Autodesk Inventor part; units mm, degrees
ref_plane "YZ Plane" through (0, 0, 0) normal (1, 0, 0) x (0, 1, 0)
ref_plane "XY Plane" through (0, 0, 0) normal (0, 0, 1) x (1, 0, 0)
sketch "Sketch1" plane through (0, 0, 0) normal (0, 0, 1) x (1, 0, 0)
  circle A0 centre (0, 0) radius 2.159
  dimension "d0" = 4.318
extrude "Extrusion1" add sketch "Sketch1" along normal blind 8.128
sketch "Sketch2" plane through (0, 0, 0) normal (0, 0, -1) x (-1, 0, 0)
  circle A0 centre (0, 0) radius 2.159
  circle A1 centre (0, 0) radius 1.4986
  dimension "d3" = 2.9972
extrude "Extrusion2" cut sketch "Sketch2" against normal blind 6.096
sketch "Sketch3" plane through (0, 0, 0) normal (0, 1, 0) x (-1, 0, 0)
  line L0 (-2.159, 8.128) -> (2.159, 8.128)
  line L1 (0, -2.8448) -> (0, 17.0688)
  line L2 (2.159, 8.128) -> (0, 8.128)
  line L3 (0, 8.128) -> (0, 14.478)
  line L4 (2.159, 6.096) -> (-2.159, 6.096)
  line L5 (-2.159, 8.128) -> (2.159, 8.128)
  line L6 (2.159, 6.096) -> (2.159, 8.128)
  line L7 (-1.4986, 0) -> (1.4986, 0)
  line L8 (0, 14.478) -> (1.9685, 14.478)
  line L9 (1.9685, 14.478) -> (2.159, 8.128)
  point P0 (0, 0)
  dimension "d22" = 8.128
  dimension "d23" = 6.096
  dimension "d24" = 6.35
  dimension "d25" = 1.9685
revolve "Revolution1" add sketch "Sketch3" angle 360 about axis through (0, 0, -10) along (0, 0, 1) contours L1 L8 L9 L0
hole "Hole1" at (0, 0, 14.478) direction (0, 0, -1) diameter 0.8382 end through all
ref_plane "Work Plane1" through (0, 2.159, 0) normal (0, 1, 0) x (-1, 0, 0)
sketch "Sketch5" plane through (0, 2.159, 0) normal (0, 1, 0) x (-1, 0, 0)
  line L0 (2.159, 6.096) -> (-2.159, 6.096)
  line L1 (-2.159, 8.128) -> (2.159, 8.128)
  line L2 (0, -2.8956) -> (0, 17.3736)
  line L3 (0, 8.128) -> (0, 6.096)
  point P0 (0, 0)
  point P1 (0, 7.112)
hole "Hole2" at (0, 2.159, 7.112) direction (0, -1, 0) diameter 1.1938 end through all
equation "\"d25\" = 0.5 * d0 - 0.03 * d6"
properties part number "Tool_Mount_Luer_Adapter_Force" material "Acetal Resin, White"
Work out the finished part from the listing and answer in its coordinate system (mm). A direction names the side the tool comes from. Coordinates: 2 decimals unless noted, no trailing zeros. Order: outer loops, then holes, each group sorted by start corner. A loop starts at its lowest first (then second) coordinate and runs counter-clockwise, first axis right, second up. Notation, with made-up numbers: (-28.75, -13) - (3.25, -13) arc R13 cw to (3.25, 12) - close; hole circle Ø5 at (-28.5, -39.5). An arc over 180 degrees is marked (long way). Put each result on its own line as item: value. Start each with the question number.
1) Find section C-C (z = 12.75). Give the vertices of the cut face in (x, y).
2) Find section A-A (x = 0). Give the vertices of the cut face in (y, z).
3) For a pull along X with two mould halves and no side action, classify faces 1 (the flat face through (-0.9, -1.4, 6.096)), 2 (the cylindrical face through (0.41, 0.09, 3.3)), 3 (the cylindrical face through (0.996, 1.915, 7.098)) as released by +X, released by -X, zero draft, split by the parting line, or undercut.
4) Find section B-B (y = 0). Give the vertices of the cut face in (x, z).
5) For faces 4 (the conical face through (1.639, -1.257, 11.259)), 5 (the flat face through (-0.41, 0.41, 14.478)), 6 (the cylindrical face through (-1.43, 0.45, 3.01)), determine the directions among +Z, -Z, +X, -X, +Y, -Y from which every point of the face is accessible in a straight line to the end or side of a thin tool.
6) Flat-ended cylindrical pins translate along their axes: pin 1 (1 mm diameter, centred on x = 0, z = 7.112, fed in from -Y); pin 2 (1.5 mm diameter, centred on y = 1.5, z = 6, fed in from -X); pin 3 (2 mm diameter, centred on x = -1.5, z = 12, fed in from +Y). Find the tip coordinate at first contact, or state that the pin passes through.
7) Find the intervals of material crossed by line 1 (Y direction, x = 0, z = 3.75); line 2 (Z direction, x = 0, y = -0.75); line 3 (X direction, y = 0, z = 9), in increasing order. Write a range as from..to.
8) Find section D-D (z = 9.5). Give the vertices of the cut face in (x, y).
Results list:
1. outline: circle Ø4.04 at (0, 0); hole circle Ø0.84 at (0, 0)
2. outline: (-2.16, 6.1) - (-1.5, 6.1) - (-1.5, 0) - (-0.42, 0) - (-0.42, 6.52) - (-2.16, 6.52) - close; (-2.16, 7.71) - (-0.42, 7.71) - (-0.42, 14.48) - (-1.97, 14.48) - (-2.16, 8.13) - close; (0.42, 0) - (1.5, 0) - (1.5, 6.1) - (2.16, 6.1) - (2.16, 6.52) - (0.42, 6.52) - close; (0.42, 7.71) - (2.16, 7.71) - (2.16, 8.13) - (1.97, 14.48) - (0.42, 14.48) - close
3. face 1: zero draft
3. face 2: undercut
3. face 3: split by the parting line
4. outline: (-2.16, 6.1) - (-1.5, 6.1) - (-1.5, 0) - (-0.42, 0) - (-0.42, 6.69) arc R0.6 cw to (-0.42, 7.54) - (-0.42, 14.48) - (-1.97, 14.48) - (-2.16, 8.13) - close; (0.42, 0) - (1.5, 0) - (1.5, 6.1) - (2.16, 6.1) - (2.16, 8.13) - (1.97, 14.48) - (0.42, 14.48) - (0.42, 7.54) arc R0.6 cw to (0.42, 6.69) - close
5. face 4: +Z
5. face 5: +Z, +X, -X, +Y, -Y
5. face 6: -Z
6. pin 1: passes through
6. pin 2: stops at x = -2.02
6. pin 3: stops at y = 1.98
7. line 1: y = -1.5..-0.42, 0.42..1.5
7. line 2: z = 0..6.52, 7.71..14.48
7. line 3: x = -2.13..-0.42, 0.42..2.13
8. outline: circle Ø4.24 at (0, 0); hole circle Ø0.84 at (0, 0)
